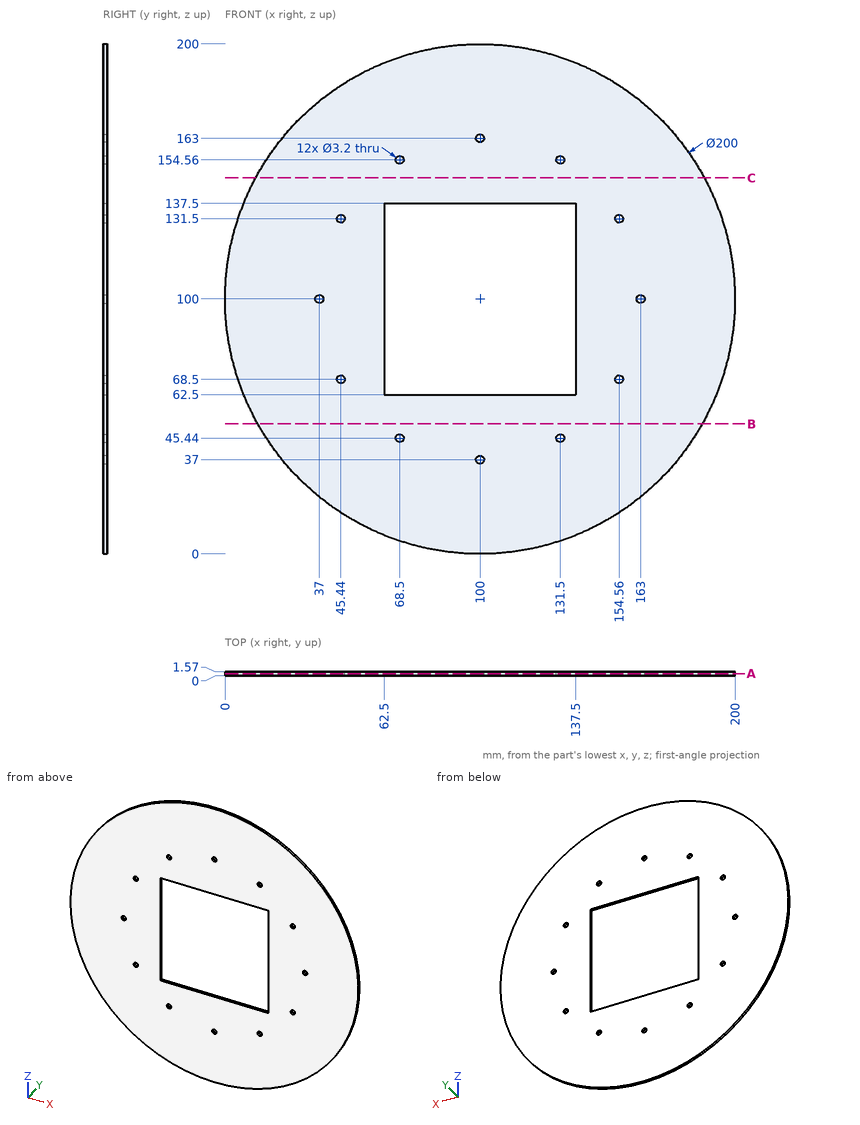
Geometry check sheet. Reference: drawing and pictorial views, mm from the part's lowest x, y, z. Round coordinates to 2 decimals unless told otherwise and drop trailing zeros. Loops run counter-clockwise (first coordinate to the right, second up) from the corner with the lowest first, then second, coordinate; pieces in that order, holes last. Notation, with made-up numbers: (-24.5, 55) - (29.5, 55) arc R19 ccw to (29.5, 89) - close; hole circle Ø1 at (24.25, -24). An arc over 180 degrees is marked (long way). Answer as CSV lines item,"result".
(1) Cross-section at B-B, the plane z = 51. Enter the section's corners in (x, y).
Output values:
outline,"(12.83, 0) - (187.17, 0) - (187.17, 1.57) - (12.83, 1.57) - close"
(2) Material ranges on line 1 along Z through (x, y) = (68.5, 0.45); line 2 along Z through (x, y) = (106, 1.25), recorded low to high.
Output values:
line 1,"z = 5.09 to 43.84, 47.04 to 62.5, 137.5 to 152.96, 156.16 to 194.91"
line 2,"z = 0.18 to 62.5, 137.5 to 199.82"
(3) Cross-section at C-C, the plane z = 147.5. Enter the section's corners in (x, y).
Output values:
outline,"(12, 0) - (188, 0) - (188, 1.57) - (12, 1.57) - close"
(4) Cross-section at A-A, the plane y = 0.9. Give the number of separate pieces and of enclosed holes in the cut face, and give its area (3 significant figures).
Output values:
separate pieces,"1"
enclosed holes,"13"
area,"25,700 mm²"
